Could you check a few things on this drawing? It's one solid part, dimensions in mm from its lowest x, y, z. Coordinates: 2 decimals unless noted, no trailing zeros. Write each loop counter-clockwise with the first axis right and the second up, starting at its lowest first coordinate (ties: lowest second). Pieces come first, ordered by that corner, then holes. Notation, with made-up numbers: (9, 77) - (66, 77) arc R26 ccw to (66, 91) - close; hole circle Ø9 at (53, 39.25). An arc over 180 degrees is marked (long way). Use one line per item in the form item = value. Start each with the question number.
(1) For pin 1 Ø8 at (x, z) = (74.3, 142.6) entering from -Y (1 decimal); pin 2 Ø2 at (y, z) = (5, 26) entering from -X; pin 3 Ø6.5 at (x, z) = (6, 74.3) entering from -Y (1 decimal), each with a flat end and sliding along its axis, tell me the tip position at first contact or that it passes through.
(2) If we section it at D-D on z = 90.5: Please give me the cut outline in (x, y), then the cut area to 3 significant figures.
(3) If I drill on probe 1 along Z at (x, y) = (74.3, 3); probe 2 along Z at (x, y) = (74.5, 1.5); probe 3 along Z at (x, y) = (121.5, 3.75) (1 decimal), over which ranges is the centre line in solid material (lowest first)? Write a range as from..to.
(4) If we section it at C-C on y = 7: Please give me the cut outline in (x, z).
(5) If we section it at A-A on z = 74.3: Please give me the cut outline in (x, y) (1 decimal).
(6) Thinking about a two-plate mould opening in Z: for the marked faces 1 and 2, which applies, pulls with the +Z half, pulls with the -Z half, needs draft (parallel to the pull), parting line crosses it, or undercut?
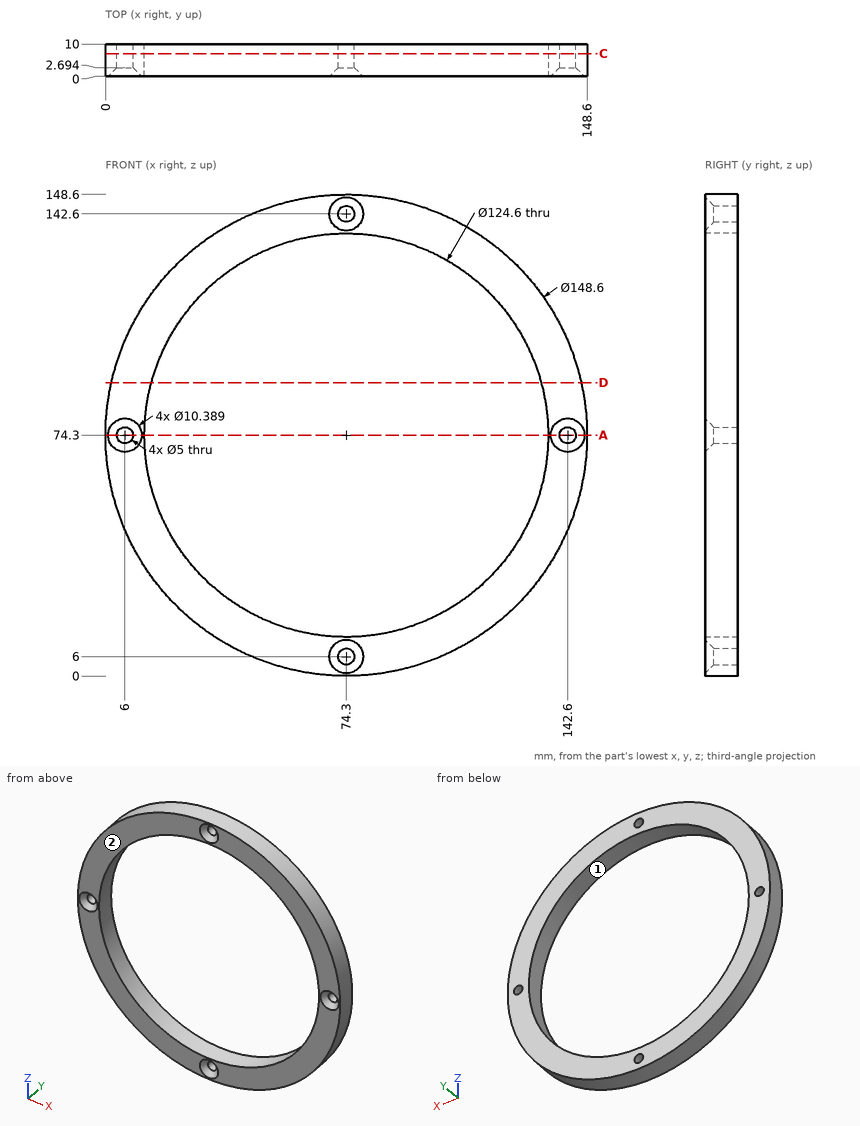
Reported:
q1.pin_1 = 1.2
q1.pin_2 = 17
q1.pin_3 = 1.9
q2.outline = (1.79, 0) - (14.14, 0) - (14.14, 10) - (1.79, 10) - close; (134.46, 0) - (146.81, 0) - (146.81, 10) - (134.46, 10) - close
q2.area = 247 mm2
q3.probe_1 = 0..3.5, 8.5..12, 136.6..140.1, 145.1..148.6
q3.probe_2 = 0..2.31, 9.69..12, 136.6..138.91, 146.29..148.6
q3.probe_3 = 16.9..33.6, 115..131.7
q4.outline = circle Ø148.6 at (74.3, 74.3); hole circle Ø5 at (6, 74.3); hole circle Ø124.6 at (74.3, 74.3); hole circle Ø5 at (74.3, 6); hole circle Ø5 at (74.3, 142.6); hole circle Ø5 at (142.6, 74.3)
q5.outline = (0, 0) - (0.8, 0) - (3.5, 2.7) - (3.5, 10) - (0, 10) - close; (8.5, 2.7) - (11.2, 0) - (12, 0) - (12, 10) - (8.5, 10) - close; (136.6, 0) - (137.4, 0) - (140.1, 2.7) - (140.1, 10) - (136.6, 10) - close; (145.1, 2.7) - (147.8, 0) - (148.6, 0) - (148.6, 10) - (145.1, 10) - close
q6.face_1 = undercut
q6.face_2 = needs draft
